Build history of the part. All positions in model axes, mm. A direction names the side the tool comes from. Give positions to 0.01 mm unless a question says otherwise; leave off trailing zeros. Loops run counter-clockwise (first coordinate to the right, second up) from the corner with the lowest first, then second, coordinate; pieces in that order, holes last. Notation, with made-up numbers: (76, 82.5) -> (91, 82.5) arc R35 cw to (91, 120.5) -> close; hole circle Ø7 at (58.5, 61). An arc over 180 degrees is marked (long way). One line per question, with ' | ' between items. Start each with the question number.
(1) Drill centre lines: L1, parallel to X at y = -159, z = -15; L2, parallel to Y at x = 266.35, z = -15; L3, parallel to X at y = 5, z = 5. Where is each one in solid material? Low to high. Write a range as from..to.
(2) Slice it at C-C, the plane x = -164. Write the cut outline in (y, z), then the cut area to 3 significant figures.
(3) Flat gauge pins, fed straight in: pin 1 Ø9 at (y, z) = (169, -17.5) entering from +X; pin 2 Ø24 at (x, z) = (-238.5, -17.5) entering from -Y; pin 3 Ø5 at (x, y) = (45, 103.5) entering from +Z. Where does each tip first touch, or does it go through?
(4) Slice it at A-A, the plane x = -37. Write the cut outline in (y, z), then the cut area to 3 significant figures.
(5) Mould opens along Y. For faces 6 (the face through (253, 27.13, -15)), 7 (the face through (253, 25.13, -15)), 8 (the face through (18, 170, -30)) say: pulls with the +Y half, pulls with the -Y half, needs draft (parallel to the pull), parting line crosses it, or undercut.
(6) Slice it at B-B, the plane y = 72. Write the cut outline in (x, z), then the cut area to 3 significant figures.
(7) 3-axis set-ups, long thin cutter, end or side, ignore diameter. For faces 1 (the face through (4, -200.37, 17)), 2 (the face through (8, 155.13, -15)), 3 (the face through (310.212, 15, 17)), 4 (the face through (253, -2.87, -15)), 5 (the face through (265.462, 9, -15)): which of +Z, -Z, +X, -X, +Y, -Y reach the whole face in a straight line?
```python
from build123d import *

# Parameters (mm, degrees)
SKETCH_1_W          = 612
SKETCH_1_H          = 425
EXTRUDE_1_DEPTH     = 2
SKETCH_2_W          = 100
SKETCH_2_H          = 32
EXTRUDE_2_DEPTH     = 2
SKETCH_3_W          = 32
SKETCH_3_H          = 100
EXTRUDE_3_DEPTH     = 2
SKETCH_4_W          = 100
SKETCH_4_H          = 32
EXTRUDE_4_DEPTH     = 2
SKETCH_5_W          = 32
SKETCH_5_H          = 100
EXTRUDE_5_DEPTH     = 2
SKETCH_6_W          = 30
SKETCH_6_H          = 30
SKETCH_6_W_2        = 26
SKETCH_6_H_2        = 26
EXTRUDE_6_DEPTH     = 30
SKETCH_7_W          = 30
SKETCH_7_H          = 30
SKETCH_7_W_2        = 26
SKETCH_7_H_2        = 26
EXTRUDE_7_DEPTH     = 30
SKETCH_8_R          = 2
CUT_EXTRUDE_1_DEPTH = 388.5
SKETCH_9_R          = 2
CUT_EXTRUDE_2_DEPTH = 572.25


with BuildPart() as part:
    # 草圖1 → 填料-伸長1 (new body)
    with BuildSketch(Plane.XY):
        with Locations((4.21177851, 12.129893238)):
            Rectangle(SKETCH_1_W, SKETCH_1_H)
    extrude(amount=EXTRUDE_1_DEPTH)

    # 草圖2 → 填料-伸長2 (add)
    with BuildSketch(Plane.XZ.offset(200.370106762)):
        with Locations((4.21177851, 16)):
            Rectangle(SKETCH_2_W, SKETCH_2_H)
    extrude(amount=EXTRUDE_2_DEPTH)

    # 草圖3 → 填料-伸長3 (add)
    with BuildSketch(Plane.ZY.offset(301.78822149)):
        with Locations((16, 14.629893238)):
            Rectangle(SKETCH_3_W, SKETCH_3_H)
    extrude(amount=EXTRUDE_3_DEPTH)

    # 草圖4 → 填料-伸長4 (add)
    with BuildSketch(Plane(origin=(0, 224.629893238, 0), x_dir=(1, 0, 0), z_dir=(0, 1, 0))):
        with Locations((4.21177851, -16)):
            Rectangle(SKETCH_4_W, SKETCH_4_H)
    extrude(amount=EXTRUDE_4_DEPTH)

    # 草圖5 → 填料-伸長5 (add)
    with BuildSketch(Plane(origin=(310.21177851, 0, 0), x_dir=(0, 0, -1), z_dir=(1, 0, 0))):
        with Locations((-16, 14.629893238)):
            Rectangle(SKETCH_5_W, SKETCH_5_H)
    extrude(amount=EXTRUDE_5_DEPTH)

    # 草圖6 → 填料-伸長6 (add)
    with BuildSketch(Plane(origin=(0, 0, 0), x_dir=(-1, 0, 0), z_dir=(0, 0, -1))):
        with Locations((-252.46177851, 12.129893238)):
            Rectangle(SKETCH_6_W, SKETCH_6_H)
        with Locations((-252.46177851, 12.129893238)):
            Rectangle(SKETCH_6_W_2, SKETCH_6_H_2, mode=Mode.SUBTRACT)
        with Locations((244.03822149, 12.129893238)):
            Rectangle(SKETCH_6_W, SKETCH_6_H)
        with Locations((244.03822149, 12.129893238)):
            Rectangle(SKETCH_6_W_2, SKETCH_6_H_2, mode=Mode.SUBTRACT)
    extrude(amount=EXTRUDE_6_DEPTH)

    # 草圖7 → 填料-伸長7 (add)
    with BuildSketch(Plane(origin=(0, 0, 0), x_dir=(-1, 0, 0), z_dir=(0, 0, -1))):
        with Locations((-4.21177851, -145.870106762)):
            Rectangle(SKETCH_7_W, SKETCH_7_H)
        with Locations((-4.21177851, -145.870106762)):
            Rectangle(SKETCH_7_W_2, SKETCH_7_H_2, mode=Mode.SUBTRACT)
        with Locations((-4.21177851, 170.129893238)):
            Rectangle(SKETCH_7_W, SKETCH_7_H)
        with Locations((-4.21177851, 170.129893238)):
            Rectangle(SKETCH_7_W_2, SKETCH_7_H_2, mode=Mode.SUBTRACT)
    extrude(amount=EXTRUDE_7_DEPTH)

    # 草圖8 → 除料-伸長1 (cut, through all)
    with BuildSketch(Plane(origin=(0, 185.129893238, 0), x_dir=(1, 0, 0), z_dir=(0, 1, 0))):
        with Locations((4.21177851, 15)):
            Circle(SKETCH_8_R)
    extrude(amount=-CUT_EXTRUDE_1_DEPTH, mode=Mode.SUBTRACT)

    # 草圖9 → 除料-伸長2 (cut, through all)
    with BuildSketch(Plane.ZY.offset(259.03822149)):
        with Locations((-15, 12.129893238)):
            Circle(SKETCH_9_R)
    extrude(amount=-CUT_EXTRUDE_2_DEPTH, mode=Mode.SUBTRACT)


solid = part.part
```
Final values:
1) L1: -10.79..2.21, 6.21..19.21 | L2: -2.87..10.13, 14.13..27.13 | L3: -303.79..-301.79, 310.21..312.21
2) outline: (-200.37, 0) -> (224.63, 0) -> (224.63, 2) -> (-200.37, 2) -> close | area: 850 mm2
3) pin 1: x = 19.21 | pin 2: y = -2.87 | pin 3: z = 2
4) outline: (-202.37, 0) -> (226.63, 0) -> (226.63, 32) -> (224.63, 32) -> (224.63, 2) -> (-200.37, 2) -> (-200.37, 32) -> (-202.37, 32) -> close | area: 978 mm2
5) face 6: pulls with the +Y half | face 7: undercut | face 8: needs draft
6) outline: (-301.79, 0) -> (310.21, 0) -> (310.21, 2) -> (-301.79, 2) -> close | area: 1,220 mm2
7) face 1: +Z, +X, -X | face 2: -Z, +X, -X | face 3: +Z, +Y, -Y | face 4: -Z, +X, -X, -Y | face 5: -Z
